from build123d import *

# Parameters (mm, degrees)
SKETCH_1_W          = 68
SKETCH_1_H          = 40
SKETCH_1_R          = 2.5
EXTRUDE_1_DEPTH     = 6
SKETCH_3_W          = 68
SKETCH_3_H          = 6
EXTRUDE_2_DEPTH     = 50
CUT_EXTRUDE_1_REACH = 8
SKETCH_4_R          = 8
SKETCH_4_R_2        = 3


with BuildPart() as part:
    # 草图1 → 凸台-拉伸1 (new body)
    with BuildSketch(Plane(origin=(0, 0, 0), x_dir=(1, 0, 0), z_dir=(0, 1, 0))):
        with Locations((0, 20)):
            Rectangle(SKETCH_1_W, SKETCH_1_H)
        with Locations((-27.5, 25)):
            Circle(SKETCH_1_R, mode=Mode.SUBTRACT)
        with Locations((27.5, 25)):
            Circle(SKETCH_1_R, mode=Mode.SUBTRACT)
        with Locations((-27.5, 5)):
            Circle(SKETCH_1_R, mode=Mode.SUBTRACT)
        with Locations((27.5, 5)):
            Circle(SKETCH_1_R, mode=Mode.SUBTRACT)
    extrude(amount=EXTRUDE_1_DEPTH)

    # 草图3 → 凸台-拉伸2 (add)
    with BuildSketch(Plane(origin=(0, 6, 0), x_dir=(1, 0, 0), z_dir=(0, 1, 0))):
        with Locations((0, 37)):
            Rectangle(SKETCH_3_W, SKETCH_3_H)
    extrude(amount=-EXTRUDE_2_DEPTH)

    # 草图4 → 切除-拉伸1 (cut, up to next)
    with BuildSketch(Plane.XY.offset(-34), mode=Mode.PRIVATE) as cut_extrude_1_sk1:
        with Locations((-1, -18)):
            Circle(SKETCH_4_R)
    cut_extrude_1_tool1 = extrude(cut_extrude_1_sk1.sketch, amount=-CUT_EXTRUDE_1_REACH, mode=Mode.PRIVATE) & part.part
    add(cut_extrude_1_tool1.solids().sort_by_distance((-1, -18, -34))[0], mode=Mode.SUBTRACT)
    # 草图4 → 切除-拉伸1 (cut, up to next)
    with BuildSketch(Plane.XY.offset(-34), mode=Mode.PRIVATE) as cut_extrude_1_sk2:
        with Locations((23, -18)):
            Circle(SKETCH_4_R_2)
    cut_extrude_1_tool2 = extrude(cut_extrude_1_sk2.sketch, amount=-CUT_EXTRUDE_1_REACH, mode=Mode.PRIVATE) & part.part
    add(cut_extrude_1_tool2.solids().sort_by_distance((23, -18, -34))[0], mode=Mode.SUBTRACT)
    # 草图4 → 切除-拉伸1 (cut, up to next)
    with BuildSketch(Plane.XY.offset(-34), mode=Mode.PRIVATE) as cut_extrude_1_sk3:
        with Locations((-25, -18)):
            Circle(SKETCH_4_R_2)
    cut_extrude_1_tool3 = extrude(cut_extrude_1_sk3.sketch, amount=-CUT_EXTRUDE_1_REACH, mode=Mode.PRIVATE) & part.part
    add(cut_extrude_1_tool3.solids().sort_by_distance((-25, -18, -34))[0], mode=Mode.SUBTRACT)


solid = part.part
Part model, mm, in its own coordinate system. A direction names the side the tool comes from. Round coordinates to 2 decimals unless told otherwise and drop trailing zeros. Order: outer loops, then holes, each group sorted by start corner. A loop starts at its lowest first (then second) coordinate and runs counter-clockwise, first axis right, second up. Notation, with made-up numbers: (70.25, 48.5) -> (103.25, 48.5) arc R24 cw to (103.25, 61.5) -> close; hole circle Ø5 at (-29.75, 52). An arc over 180 degrees is marked (long way). Put each result on its own line as item: value.
Q1. Band-saw the part on D-D (y = 2.5). Give the cut face in (x, z).
From the geometry:
outline: (-34, -40) -> (34, -40) -> (34, 0) -> (-34, 0) -> close; hole circle Ø5 at (-27.5, -25); hole circle Ø5 at (-27.5, -5); hole circle Ø5 at (27.5, -25); hole circle Ø5 at (27.5, -5)
Q2. Band-saw the part on A-A (x = 23). Give the cut face in (y, z), and give its area (3 significant figures).
From the geometry:
outline: (-44, -40) -> (-21, -40) -> (-21, -34) -> (-44, -34) -> close; (-15, -40) -> (6, -40) -> (6, 0) -> (0, 0) -> (0, -34) -> (-15, -34) -> close
area: 468 mm2
Q3. Band-saw the part on B-B (y = -18). Give the cut face in (x, z), and give its area (3 significant figures).
From the geometry:
outline: (-34, -40) -> (-28, -40) -> (-28, -34) -> (-34, -34) -> close; (-22, -40) -> (-9, -40) -> (-9, -34) -> (-22, -34) -> close; (7, -40) -> (20, -40) -> (20, -34) -> (7, -34) -> close; (26, -40) -> (34, -40) -> (34, -34) -> (26, -34) -> close
area: 240 mm2
Q4. Tool access for faces 1 (the face through (0, 0, -17)), 2 (the face through (0, -44, -37)): list every direction of +Z, -Z, +X, -X, +Y, -Y with a clear straight run to the whole face (end or side of a thin tool).
From the geometry:
face 1: +Z, +X, -X, -Y
face 2: +Z, -Z, +X, -X, -Y
Q5. Wall check: line 1 (Z direction, x = 27.5, y = 4.65); line 2 (Y direction, x = -25, z = -38.6); line 3 (Y direction, x = 6.5, z = -1.5). Give the ranges that are in metal, low to high. Write a range as [from, to].
From the geometry:
line 1: z = [-40, -27.5], [-22.5, -7.5], [-2.5, 0]
line 2: y = [-44, -21], [-15, 6]
line 3: y = [0, 6]
Q6. Pin check, flat tips, straight feed: pin 1 Ø1.5 at (x, z) = (-20, -24) entering from -Y; pin 2 Ø6 at (x, z) = (27.5, -5) entering from +Y; pin 3 Ø9.5 at (x, y) = (23, -18) entering from +Z. Stop position of each tip, or through.
From the geometry:
pin 1: stops at y = 0
pin 2: stops at y = 6
pin 3: stops at z = -34
Q7. Pull direction X, two halves, no side cores. Call faces 3 (the face through (26, 3, -7)), 4 (the face through (-34, -10, -35)), 5 (the face through (0, -27, -34)): pulls with the +X half, pulls with the -X half, needs draft (parallel to the pull), parting line crosses it, or undercut.
From the geometry:
face 3: undercut
face 4: pulls with the -X half
face 5: needs draft
Q8. Band-saw the part on C-C (z = -25). Give the cut face in (x, y), and give its area (3 significant figures).
From the geometry:
outline: (-34, 0) -> (-30, 0) -> (-30, 6) -> (-34, 6) -> close; (-25, 0) -> (25, 0) -> (25, 6) -> (-25, 6) -> close; (30, 0) -> (34, 0) -> (34, 6) -> (30, 6) -> close
area: 348 mm2
